Part model, mm, in its own coordinate system. A direction names the side the tool comes from. Give positions to 0.01 mm unless a question says otherwise; leave off trailing zeros. Write each loop counter-clockwise with the first axis right and the second up, starting at its lowest first coordinate (ties: lowest second). Pieces come first, ordered by that corner, then holes.
from build123d import *

# Parameters (mm, degrees)
SKETCH_1_W                       = 120
SKETCH_1_H                       = 80
DECK_120X80X3_DEPTH              = 3
FRAME_RIB_START                  = 3
SKETCH_2_W                       = 8.4
SKETCH_2_H                       = 9.4
FRAME_RIB_DEPTH                  = 7.5
EXTRUDE_START                    = 3
SKETCH_3_W                       = 8.4
SKETCH_3_H                       = 9.4
EXTRUDE_3_DEPTH                  = 7.5
MOUNT_UPRIGHT_START              = 10.5
SKETCH_4_W                       = 7
SKETCH_4_H                       = 2.5
MOUNT_UPRIGHT_DEPTH              = 17
EXTRUDE_START_2                  = 10.5
SKETCH_5_W                       = 7
SKETCH_5_H                       = 2.5
EXTRUDE_5_DEPTH                  = 17
MOUNT_LOWER_BEAM_START           = 7.5
SKETCH_6_W                       = 38
SKETCH_6_H                       = 2.5
MOUNT_LOWER_BEAM_DEPTH           = 3.4
MOUNT_UPPER_BEAM_START           = 24.1
SKETCH_7_W                       = 38
SKETCH_7_H                       = 2.5
MOUNT_UPPER_BEAM_DEPTH           = 3.4
SERVO_EAR_ADJUSTABLE_SLOTS_START = -46.5
SKETCH_8_W                       = 3.4
SKETCH_8_H                       = 2.5
SERVO_EAR_ADJUSTABLE_SLOTS_DEPTH = 4
SKETCH_9_W                       = 8.4
SKETCH_9_H                       = 9.4
EXTRUDE_8_DEPTH                  = 7.5
SKETCH_10_W                      = 8.4
SKETCH_10_H                      = 9.4
EXTRUDE_9_DEPTH                  = 7.5
SKETCH_11_W                      = 7
SKETCH_11_H                      = 2.5
EXTRUDE_10_DEPTH                 = 17
SKETCH_12_W                      = 7
SKETCH_12_H                      = 2.5
EXTRUDE_11_DEPTH                 = 17
EXTRUDE_START_3                  = 7.5
SKETCH_13_W                      = 38
SKETCH_13_H                      = 2.5
EXTRUDE_12_DEPTH                 = 3.4
EXTRUDE_START_4                  = 24.1
SKETCH_14_W                      = 38
SKETCH_14_H                      = 2.5
EXTRUDE_13_DEPTH                 = 3.4
CUT_EXTRUDE_START                = 42.5
SKETCH_15_W                      = 3.4
SKETCH_15_H                      = 2.5
CUT_EXTRUDE_2_DEPTH              = 4
SKETCH_16_W                      = 8.4
SKETCH_16_H                      = 9.4
EXTRUDE_14_DEPTH                 = 7.5
SKETCH_17_W                      = 8.4
SKETCH_17_H                      = 9.4
EXTRUDE_15_DEPTH                 = 7.5
SKETCH_18_W                      = 7
SKETCH_18_H                      = 2.5
EXTRUDE_16_DEPTH                 = 17
SKETCH_19_W                      = 7
SKETCH_19_H                      = 2.5
EXTRUDE_17_DEPTH                 = 17
SKETCH_20_W                      = 38
SKETCH_20_H                      = 2.5
EXTRUDE_18_DEPTH                 = 3.4
SKETCH_21_W                      = 38
SKETCH_21_H                      = 2.5
EXTRUDE_19_DEPTH                 = 3.4
CUT_EXTRUDE_START_2              = -46.5
SKETCH_22_W                      = 3.4
SKETCH_22_H                      = 2.5
CUT_EXTRUDE_3_DEPTH              = 4
SKETCH_23_W                      = 8.4
SKETCH_23_H                      = 9.4
EXTRUDE_20_DEPTH                 = 7.5
SKETCH_24_W                      = 8.4
SKETCH_24_H                      = 9.4
EXTRUDE_21_DEPTH                 = 7.5
SKETCH_25_W                      = 7
SKETCH_25_H                      = 2.5
EXTRUDE_22_DEPTH                 = 17
SKETCH_26_W                      = 7
SKETCH_26_H                      = 2.5
EXTRUDE_23_DEPTH                 = 17
SKETCH_27_W                      = 38
SKETCH_27_H                      = 2.5
EXTRUDE_24_DEPTH                 = 3.4
SKETCH_28_W                      = 38
SKETCH_28_H                      = 2.5
EXTRUDE_25_DEPTH                 = 3.4
SKETCH_29_W                      = 3.4
SKETCH_29_H                      = 2.5
CUT_EXTRUDE_4_DEPTH              = 4
M3_DECK_MOUNTING_HOLES_START     = -0.1
SKETCH_30_R                      = 1.7
M3_DECK_MOUNTING_HOLES_DEPTH     = 3.2
PCB_SCREW_ACCESS_START           = -0.1
SKETCH_31_W                      = 3.8
SKETCH_31_H                      = 2.6
PCB_SCREW_ACCESS_DEPTH           = 3.2


with BuildPart() as part:
    # 草图1 → Deck_120x80x3 (new body)
    with BuildSketch(Plane.XY):
        Rectangle(SKETCH_1_W, SKETCH_1_H)
    extrude(amount=DECK_120X80X3_DEPTH)

    # 草图2 → Frame_rib (add)
    with BuildSketch(Plane.XY.offset(FRAME_RIB_START)):
        with Locations((-63.45, -40.5)):
            Rectangle(SKETCH_2_W, SKETCH_2_H)
    extrude(amount=FRAME_RIB_DEPTH)

    # 草图3 → 凸台-拉伸3 (add)
    with BuildSketch(Plane.XY.offset(EXTRUDE_START)):
        with Locations((-33.85, -40.5)):
            Rectangle(SKETCH_3_W, SKETCH_3_H)
    extrude(amount=EXTRUDE_3_DEPTH)

    # 草图4 → Mount_upright (add)
    with BuildSketch(Plane.XY.offset(MOUNT_UPRIGHT_START)):
        with Locations((-64.15, -44.5)):
            Rectangle(SKETCH_4_W, SKETCH_4_H)
    extrude(amount=MOUNT_UPRIGHT_DEPTH)

    # 草图5 → 凸台-拉伸5 (add)
    with BuildSketch(Plane.XY.offset(EXTRUDE_START_2)):
        with Locations((-33.15, -44.5)):
            Rectangle(SKETCH_5_W, SKETCH_5_H)
    extrude(amount=EXTRUDE_5_DEPTH)

    # 草图6 → Mount_lower_beam (add)
    with BuildSketch(Plane.XY.offset(MOUNT_LOWER_BEAM_START)):
        with Locations((-48.65, -44.5)):
            Rectangle(SKETCH_6_W, SKETCH_6_H)
    extrude(amount=MOUNT_LOWER_BEAM_DEPTH)

    # 草图7 → Mount_upper_beam (add)
    with BuildSketch(Plane.XY.offset(MOUNT_UPPER_BEAM_START)):
        with Locations((-48.65, -44.5)):
            Rectangle(SKETCH_7_W, SKETCH_7_H)
    extrude(amount=MOUNT_UPPER_BEAM_DEPTH)

    # 草图8 → Servo_ear_adjustable_slots (cut)
    with BuildSketch(Plane(origin=(0, 0, 0), x_dir=(1, 0, 0), z_dir=(0, 1, 0)).offset(SERVO_EAR_ADJUSTABLE_SLOTS_START)):
        with Locations((-62.5, -17.5)):
            Rectangle(SKETCH_8_W, SKETCH_8_H)
        with Locations((-34.8, -17.5)):
            Rectangle(SKETCH_8_W, SKETCH_8_H)
    extrude(amount=SERVO_EAR_ADJUSTABLE_SLOTS_DEPTH, mode=Mode.SUBTRACT)

    # 草图9 → 凸台-拉伸8 (add)
    with BuildSketch(Plane.XY.offset(EXTRUDE_START)):
        with Locations((-63.45, 40.5)):
            Rectangle(SKETCH_9_W, SKETCH_9_H)
    extrude(amount=EXTRUDE_8_DEPTH)

    # 草图10 → 凸台-拉伸9 (add)
    with BuildSketch(Plane.XY.offset(EXTRUDE_START)):
        with Locations((-33.85, 40.5)):
            Rectangle(SKETCH_10_W, SKETCH_10_H)
    extrude(amount=EXTRUDE_9_DEPTH)

    # 草图11 → 凸台-拉伸10 (add)
    with BuildSketch(Plane.XY.offset(EXTRUDE_START_2)):
        with Locations((-64.15, 44.5)):
            Rectangle(SKETCH_11_W, SKETCH_11_H)
    extrude(amount=EXTRUDE_10_DEPTH)

    # 草图12 → 凸台-拉伸11 (add)
    with BuildSketch(Plane.XY.offset(EXTRUDE_START_2)):
        with Locations((-33.15, 44.5)):
            Rectangle(SKETCH_12_W, SKETCH_12_H)
    extrude(amount=EXTRUDE_11_DEPTH)

    # 草图13 → 凸台-拉伸12 (add)
    with BuildSketch(Plane.XY.offset(EXTRUDE_START_3)):
        with Locations((-48.65, 44.5)):
            Rectangle(SKETCH_13_W, SKETCH_13_H)
    extrude(amount=EXTRUDE_12_DEPTH)

    # 草图14 → 凸台-拉伸13 (add)
    with BuildSketch(Plane.XY.offset(EXTRUDE_START_4)):
        with Locations((-48.65, 44.5)):
            Rectangle(SKETCH_14_W, SKETCH_14_H)
    extrude(amount=EXTRUDE_13_DEPTH)

    # 草图15 → 切除-拉伸2 (cut)
    with BuildSketch(Plane(origin=(0, 0, 0), x_dir=(1, 0, 0), z_dir=(0, 1, 0)).offset(CUT_EXTRUDE_START)):
        with Locations((-62.5, -17.5)):
            Rectangle(SKETCH_15_W, SKETCH_15_H)
        with Locations((-34.8, -17.5)):
            Rectangle(SKETCH_15_W, SKETCH_15_H)
    extrude(amount=CUT_EXTRUDE_2_DEPTH, mode=Mode.SUBTRACT)

    # 草图16 → 凸台-拉伸14 (add)
    with BuildSketch(Plane.XY.offset(EXTRUDE_START)):
        with Locations((22.55, -40.5)):
            Rectangle(SKETCH_16_W, SKETCH_16_H)
    extrude(amount=EXTRUDE_14_DEPTH)

    # 草图17 → 凸台-拉伸15 (add)
    with BuildSketch(Plane.XY.offset(EXTRUDE_START)):
        with Locations((52.15, -40.5)):
            Rectangle(SKETCH_17_W, SKETCH_17_H)
    extrude(amount=EXTRUDE_15_DEPTH)

    # 草图18 → 凸台-拉伸16 (add)
    with BuildSketch(Plane.XY.offset(EXTRUDE_START_2)):
        with Locations((21.85, -44.5)):
            Rectangle(SKETCH_18_W, SKETCH_18_H)
    extrude(amount=EXTRUDE_16_DEPTH)

    # 草图19 → 凸台-拉伸17 (add)
    with BuildSketch(Plane.XY.offset(EXTRUDE_START_2)):
        with Locations((52.85, -44.5)):
            Rectangle(SKETCH_19_W, SKETCH_19_H)
    extrude(amount=EXTRUDE_17_DEPTH)

    # 草图20 → 凸台-拉伸18 (add)
    with BuildSketch(Plane.XY.offset(EXTRUDE_START_3)):
        with Locations((37.35, -44.5)):
            Rectangle(SKETCH_20_W, SKETCH_20_H)
    extrude(amount=EXTRUDE_18_DEPTH)

    # 草图21 → 凸台-拉伸19 (add)
    with BuildSketch(Plane.XY.offset(EXTRUDE_START_4)):
        with Locations((37.35, -44.5)):
            Rectangle(SKETCH_21_W, SKETCH_21_H)
    extrude(amount=EXTRUDE_19_DEPTH)

    # 草图22 → 切除-拉伸3 (cut)
    with BuildSketch(Plane(origin=(0, 0, 0), x_dir=(1, 0, 0), z_dir=(0, 1, 0)).offset(CUT_EXTRUDE_START_2)):
        with Locations((23.5, -17.5)):
            Rectangle(SKETCH_22_W, SKETCH_22_H)
        with Locations((51.2, -17.5)):
            Rectangle(SKETCH_22_W, SKETCH_22_H)
    extrude(amount=CUT_EXTRUDE_3_DEPTH, mode=Mode.SUBTRACT)

    # 草图23 → 凸台-拉伸20 (add)
    with BuildSketch(Plane.XY.offset(EXTRUDE_START)):
        with Locations((22.55, 40.5)):
            Rectangle(SKETCH_23_W, SKETCH_23_H)
    extrude(amount=EXTRUDE_20_DEPTH)

    # 草图24 → 凸台-拉伸21 (add)
    with BuildSketch(Plane.XY.offset(EXTRUDE_START)):
        with Locations((52.15, 40.5)):
            Rectangle(SKETCH_24_W, SKETCH_24_H)
    extrude(amount=EXTRUDE_21_DEPTH)

    # 草图25 → 凸台-拉伸22 (add)
    with BuildSketch(Plane.XY.offset(EXTRUDE_START_2)):
        with Locations((21.85, 44.5)):
            Rectangle(SKETCH_25_W, SKETCH_25_H)
    extrude(amount=EXTRUDE_22_DEPTH)

    # 草图26 → 凸台-拉伸23 (add)
    with BuildSketch(Plane.XY.offset(EXTRUDE_START_2)):
        with Locations((52.85, 44.5)):
            Rectangle(SKETCH_26_W, SKETCH_26_H)
    extrude(amount=EXTRUDE_23_DEPTH)

    # 草图27 → 凸台-拉伸24 (add)
    with BuildSketch(Plane.XY.offset(EXTRUDE_START_3)):
        with Locations((37.35, 44.5)):
            Rectangle(SKETCH_27_W, SKETCH_27_H)
    extrude(amount=EXTRUDE_24_DEPTH)

    # 草图28 → 凸台-拉伸25 (add)
    with BuildSketch(Plane.XY.offset(EXTRUDE_START_4)):
        with Locations((37.35, 44.5)):
            Rectangle(SKETCH_28_W, SKETCH_28_H)
    extrude(amount=EXTRUDE_25_DEPTH)

    # 草图29 → 切除-拉伸4 (cut)
    with BuildSketch(Plane(origin=(0, 0, 0), x_dir=(1, 0, 0), z_dir=(0, 1, 0)).offset(CUT_EXTRUDE_START)):
        with Locations((23.5, -17.5)):
            Rectangle(SKETCH_29_W, SKETCH_29_H)
        with Locations((51.2, -17.5)):
            Rectangle(SKETCH_29_W, SKETCH_29_H)
    extrude(amount=CUT_EXTRUDE_4_DEPTH, mode=Mode.SUBTRACT)

    # 草图30 → M3_deck_mounting_holes (cut)
    with BuildSketch(Plane.XY.offset(M3_DECK_MOUNTING_HOLES_START)):
        with Locations((-25, -28)):
            Circle(SKETCH_30_R)
        with Locations((-25, 28)):
            Circle(SKETCH_30_R)
        with Locations((25, -28)):
            Circle(SKETCH_30_R)
        with Locations((25, 28)):
            Circle(SKETCH_30_R)
        with Locations((52, -20)):
            Circle(SKETCH_30_R)
        with Locations((52, 20)):
            Circle(SKETCH_30_R)
    extrude(amount=M3_DECK_MOUNTING_HOLES_DEPTH, mode=Mode.SUBTRACT)

    # 草图31 → PCB_screw_access (cut)
    with BuildSketch(Plane.XY.offset(PCB_SCREW_ACCESS_START)):
        with Locations((-24.3, -19.5)):
            Rectangle(SKETCH_31_W, SKETCH_31_H)
        with Locations((-24.3, 19.5)):
            Rectangle(SKETCH_31_W, SKETCH_31_H)
        with Locations((24.3, -19.5)):
            Rectangle(SKETCH_31_W, SKETCH_31_H)
        with Locations((24.3, 19.5)):
            Rectangle(SKETCH_31_W, SKETCH_31_H)
    extrude(amount=PCB_SCREW_ACCESS_DEPTH, mode=Mode.SUBTRACT)


solid = part.part
1) Saw through at B-B (z = 14.25). State how many separate pieces and enclosed holes the cut face has, and give its area (3 significant figures).
Check result:
separate pieces: 8
enclosed holes: 0
area: 140 mm2
2) Drill centre lines: L1, parallel to X at y = -20, z = 1.7; L2, parallel to Y at x = -25, z = 1.25; L3, parallel to X at y = -28, z = 1.8. Where is each one in solid material? Low to high.
Check result:
L1: x = -60 to -26.2, -22.4 to 22.4, 26.2 to 50.3, 53.7 to 60
L2: y = -40 to -29.7, -26.3 to -20.8, -18.2 to 18.2, 20.8 to 26.3, 29.7 to 40
L3: x = -60 to -26.7, -23.3 to 23.3, 26.7 to 60
3) Saw through at D-D (x = 0). Write the cut outline in (y, z).
Check result:
outline: (-40, 0) - (40, 0) - (40, 3) - (-40, 3) - close
4) 3-axis set-ups, long thin cutter, end or side, ignore diameter. For faces 4 (the flat face through (22.4, 19, 1)), 5 (the flat face through (-67.65, -42, 10)), 6 (the flat face through (-34, 35.8, 7)), 7 (the flat face through (37, 45, 24.1)): which of +Z, -Z, +X, -X, +Y, -Y reach the whole face in a straight line?
Check result:
face 4: +Z, -Z
face 5: +Z, -Z, -X, +Y, -Y
face 6: +Z, +X, -X
face 7: +Y, -Y
5) Saw through at C-C (y = 37.5). Write the cut outline in (x, z), and give its area (3 significant figures).
Check result:
outline: (-67.65, 3) - (-60, 3) - (-60, 0) - (60, 0) - (60, 3) - (56.35, 3) - (56.35, 10.5) - (47.95, 10.5) - (47.95, 3) - (26.75, 3) - (26.75, 10.5) - (18.35, 10.5) - (18.35, 3) - (-29.65, 3) - (-29.65, 10.5) - (-38.05, 10.5) - (-38.05, 3) - (-59.25, 3) - (-59.25, 10.5) - (-67.65, 10.5) - close
area: 612 mm2
6) Saw through at A-A (y = -28). Write the cut outline in (x, z).
Check result:
outline: (-60, 0) - (-26.7, 0) - (-26.7, 3) - (-60, 3) - close; (-23.3, 0) - (23.3, 0) - (23.3, 3) - (-23.3, 3) - close; (26.7, 0) - (60, 0) - (60, 3) - (26.7, 3) - close
7) Flat gauge pins, fed straight in: P1, Ø6, axis at x = 50.5, y = 39.5, coming from the +Z side; P2, Ø1.5, axis at x = 3.5, y = -8.5, coming from the +Z side; P3, Ø1.2, axis at x = -34, y = -45, coming from the -Z side. Where does each tip first touch, or does it go through?
Check result:
P1: stops at z = 10.5
P2: stops at z = 3
P3: stops at z = 3
8) Mould opens along X. For faces 1 (the flat face through (-67.65, 42, 10)), 2 (the cylindrical face through (-24.086, 29.433, 1.479)), 3 (the flat face through (37.1, -45.75, 10.7)) say: +X half, -X half, draft (parallel to the pull), parting line (faces both ways), or undercut.
Check result:
face 1: -X half
face 2: undercut
face 3: draft
